```python
from build123d import *

# Parameters (mm, degrees)
SKETCH1_W        = 42
SKETCH1_H        = 12
SKETCH1_R        = 2.5
MAIN_BOSS_DEPTH  = 10
SKETCH2_R        = 1.75
SKETCH2_R_2      = 9.5
SIDE_HOLES_DEPTH = 27.172504657
FILLET2_R        = 1.5
CHAMFER2_SIZE    = 3


with BuildPart() as part:
    # Sketch1 → main boss (new body)
    with BuildSketch(Plane(origin=(0, 0, 0), x_dir=(1, 0, 0), z_dir=(0, 1, 0))):
        Rectangle(SKETCH1_W, SKETCH1_H)
        with Locations(Location((-10, 0, 0), (0, 0, 270))):
            Circle(SKETCH1_R, mode=Mode.SUBTRACT)
        with Locations(Location((10, 0, 0), (0, 0, 90))):
            Circle(SKETCH1_R, mode=Mode.SUBTRACT)
    extrude(amount=MAIN_BOSS_DEPTH)

    # Sketch2 → side holes (cut, through all)
    with BuildSketch(Plane.XY.offset(6)):
        with Locations((-15.5, 5.5)):
            Circle(SKETCH2_R)
        with Locations(Location((15.5, 5.5, 0), (0, 0, 180))):
            Circle(SKETCH2_R)
        with Locations((0, -6.5)):
            Circle(SKETCH2_R_2)
    extrude(amount=-SIDE_HOLES_DEPTH, mode=Mode.SUBTRACT)

    # Fillet2
    fillet2_edges = [part.edges().sort_by_distance(p)[0] for p in [
        (21, 10, 0),
        (0, 10, -6),
        (-13.964101615, 0, -6),
        (13.964101615, 0, 6),
        (0, 3, -6),
        (0, 3, 6),
        (-21, 10, 0),
        (13.964101615, 0, -6),
        (21, 0, 0),
        (-13.964101615, 0, 6),
        (-21, 0, 0),
        (-21, 5, -6),
        (21, 5, -6),
        (21, 5, 6),
        (-21, 5, 6),
        (0, 10, 6),
    ]]
    fillet(fillet2_edges, radius=FILLET2_R)

    # Chamfer2
    # the kernel refuses this chamfer: 3 mm, written as the material it takes off along each edge
    with BuildSketch(Plane(origin=(-10, 0, 0), x_dir=(0, 0, 1), z_dir=(-1, 0, 0))) as chamfer2_piece_1:
        Polygon((2.5 + CHAMFER2_SIZE, 0), (2.5, CHAMFER2_SIZE), (2.5, 0), align=None)
    revolve(axis=Axis((-10, 0, 0), (0, 1, 0)), mode=Mode.SUBTRACT)
    with BuildSketch(Plane(origin=(10, 0, 0), x_dir=(0, 0, -1), z_dir=(1, 0, 0))) as chamfer2_piece_2:
        Polygon((2.5 + CHAMFER2_SIZE, 0), (2.5, CHAMFER2_SIZE), (2.5, 0), align=None)
    revolve(axis=Axis((10, 0, 0), (0, 1, 0)), mode=Mode.SUBTRACT)


solid = part.part
```
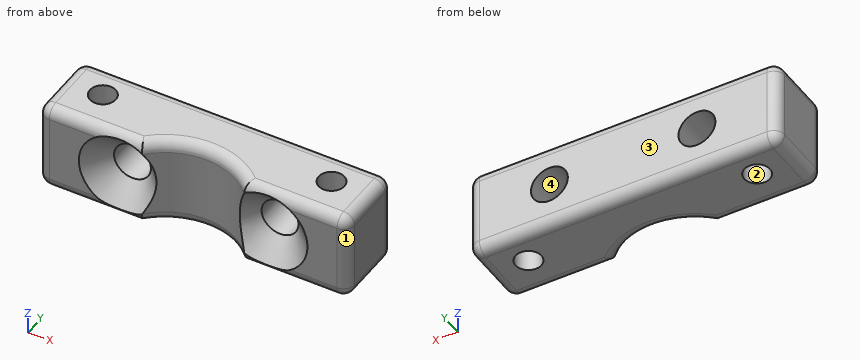
Check sheet for the modelled part. Datum: model origin and axes. Units: mm. Face numbers are marked on the shaded views. Round coordinates to 2 decimals unless told otherwise and drop trailing zeros. Order: outer loops, then holes, each group sorted by start corner. A loop starts at its lowest first (then second) coordinate and runs counter-clockwise, first axis right, second up. Notation, with made-up numbers: (30.25, -35.5) - (78.25, -35.5) arc R11 ccw to (78.25, -23.5) - close; hole circle Ø11 at (75.25, 30.5). An arc over 180 degrees is marked (long way). Write item = value, one per line.
Q1. Go/stop test with a flat-tipped pin: pin 1 (4 mm diameter, centred on x = -10, z = 0, fed in from -Y). Record where the tip stops, or that it passes through.
Computed:
pin_1 = through
Q2. Section check D-D (x = 10). Record the boundary of the cut face in (y, z).
Computed:
outline = (0.22, -5.28) arc R1.5 ccw to (1.5, -6) - (8.5, -6) arc R1.5 ccw to (10, -4.5) - (10, -2.5) - (3, -2.5) - close; (0.22, 5.28) - (3, 2.5) - (10, 2.5) - (10, 4.5) arc R1.5 ccw to (8.5, 6) - (1.5, 6) arc R1.5 ccw to start
Q3. Thickness scan on line 1 along Z through (x, y) = (10, 5.5); line 2 along Y through (x, z) = (-15.5, 3.25); line 3 along X through (y, z) = (5.25, 4). Record the ranges inside material, lowest first.
Computed:
line_1 = -6 to -2.5, 2.5 to 6
line_2 = 0 to 3.75, 7.25 to 10
line_3 = -21 to -17.23, -13.77 to 13.77, 17.23 to 21
Q4. Section check C-C (y = 8). Record the boundary of the cut face in (x, z).
Computed:
outline = (-21, -4.5) arc R1.5 ccw to (-19.5, -6) - (19.5, -6) arc R1.5 ccw to (21, -4.5) - (21, 4.5) arc R1.5 ccw to (19.5, 6) - (-19.5, 6) arc R1.5 ccw to (-21, 4.5) - close; hole circle Ø5 at (-10, 0); hole circle Ø5 at (10, 0)
Q5. Section check B-B (z = 0). Record the boundary of the cut face in (x, y).
Computed:
outline = (-21, 1.5) arc R1.5 ccw to (-19.5, 0) - (-15.5, 0) - (-12.5, 3) - (-12.5, 10) - (-19.5, 10) arc R1.5 ccw to (-21, 8.5) - close; (-7.5, 3) - (-5.64, 1.14) arc R9.5 cw to (5.64, 1.14) - (7.5, 3) - (7.5, 10) - (-7.5, 10) - close; (12.5, 3) - (15.5, 0) - (19.5, 0) arc R1.5 ccw to (21, 1.5) - (21, 8.5) arc R1.5 ccw to (19.5, 10) - (12.5, 10) - close; hole circle Ø3.5 at (-15.5, 5.5); hole circle Ø3.5 at (15.5, 5.5)
Q6. Section check A-A (y = 5.5). Record the boundary of the cut face in (x, z), and give its area (3 significant figures).
Computed:
outline = (-21, -4.5) arc R1.5 ccw to (-19.5, -6) - (-17.25, -6) - (-17.25, 6) - (-19.5, 6) arc R1.5 ccw to (-21, 4.5) - close; (-13.75, -6) - (13.75, -6) - (13.75, 6) - (-13.75, 6) - close; (17.25, -6) - (19.5, -6) arc R1.5 ccw to (21, -4.5) - (21, 4.5) arc R1.5 ccw to (19.5, 6) - (17.25, 6) - close; hole circle Ø5 at (-10, 0); hole circle Ø5 at (10, 0)
area = 379 mm^2
Q7. Draft check along Y on the marked faces 1, 2, 3 and 4. Enter one of: pulls with the +Y half, pulls with the -Y half, needs draft (parallel to the pull), parting line crosses it, or undercut.
Computed:
face_1 = pulls with the -Y half
face_2 = undercut
face_3 = pulls with the +Y half
face_4 = needs draft
